CAD build for the part. Positions are in the model's coordinates, mm. Give positions to 0.01 mm unless a question says otherwise; leave off trailing zeros. Order: outer loops, then holes, each group sorted by start corner. A loop starts at its lowest first (then second) coordinate and runs counter-clockwise, first axis right, second up. Notation, with made-up numbers: M 27.25,75.25 L 61.25,75.25 A25 ccw 61.25,102.25 Z; hole C 76.25,23 d4. An arc over 180 degrees is marked long. Put each result on its own line as item: value. Start each with the question number.
1) Cut at C-C (x = 35). Write the cut outline in (y, z).
2) Cut at D-D (y = -9.5). Write the cut outline in (x, z).
3) Drill centre lines: line 1 (Z direction, x = 22, y = -15.5); line 2 (Z direction, x = -30, y = -5); line 3 (Y direction, x = -48, z = -21.5). Where is each one in solid material? Low to high. Write a range as [from, to].
4) Cut at B-B (y = -20). Write the cut outline in (x, z), and give its area (3 significant figures).
5) Pin check, flat tips, straight feed: pin 1 (6 mm diameter, centred on x = -36.5, z = -24, fed in from +Y); pin 2 (0.8 mm diameter, centred on y = 0, z = 15, fed in from -X); pin 3 (12 mm diameter, centred on x = -32.5, y = -9, fed in from +Z). Stop position of each tip, or through.
6) Cut at A-A (z = -14). Write the cut outline in (x, y), and give its area (3 significant figures).
```python
from build123d import *

# Parameters (mm, degrees)
F0_R     = 12.7
F1_DEPTH = 38.5
F2_DEPTH = 23.11
F3_DEPTH = 6.5


with BuildPart() as f1:
    # F0 (on Top) → F1 (new body)
    with BuildSketch(Plane.XY):
        with BuildLine():
            Line((53.5, -25), (53.5, 25))
            Line((53.5, 25), (-28.5, 25))
            ThreePointArc((-28.5, 25), (-46.1776695297, 17.6776695297), (-53.5, 0))
            Line((-53.5, 0), (-53.5, -25))
            Line((-53.5, -25), (53.5, -25))
        make_face()
        with Locations((-28.5, 0)):
            Circle(F0_R, mode=Mode.SUBTRACT)
        with Locations((-28.5, 0)):
            Circle(F0_R)
        with BuildLine():
            ThreePointArc((-31.6598892386, 0.76), (-28.117338286, 3.2273936873), (-25.25, 0))
            ThreePointArc((-25.25, 0), (-28.117338286, -3.2273936873), (-31.6598892386, -0.76))
            ThreePointArc((-31.6598892386, -0.76), (-31.75, 0), (-31.6598892386, 0.76))
        make_face(mode=Mode.SUBTRACT)
        with BuildLine():
            ThreePointArc((-31.6598892386, -0.76), (-28.117338286, -3.2273936873), (-25.25, 0))
            ThreePointArc((-25.25, 0), (-28.117338286, 3.2273936873), (-31.6598892386, 0.76))
            Line((-31.6598892386, 0.76), (-31.1098892386, 0.76))
            Line((-31.1098892386, 0.76), (-31.1098892386, -0.76))
            Line((-31.1098892386, -0.76), (-31.6598892386, -0.76))
        make_face()
        with BuildLine():
            Line((-31.1098892386, 0.76), (-31.6598892386, 0.76))
            ThreePointArc((-31.6598892386, 0.76), (-31.75, 0), (-31.6598892386, -0.76))
            Line((-31.6598892386, -0.76), (-31.1098892386, -0.76))
            Line((-31.1098892386, -0.76), (-31.1098892386, 0.76))
        make_face()
    extrude(amount=-F1_DEPTH)

    # F0 (on Top) → F2 (join)
    with BuildSketch(Plane.XY):
        with BuildLine():
            ThreePointArc((-31.6598892386, -0.76), (-28.117338286, -3.2273936873), (-25.25, 0))
            ThreePointArc((-25.25, 0), (-28.117338286, 3.2273936873), (-31.6598892386, 0.76))
            Line((-31.6598892386, 0.76), (-31.1098892386, 0.76))
            Line((-31.1098892386, 0.76), (-31.1098892386, -0.76))
            Line((-31.1098892386, -0.76), (-31.6598892386, -0.76))
        make_face()
    extrude(amount=F2_DEPTH)

    # F0 (on Top) → F3 (join)
    with BuildSketch(Plane.XY):
        with Locations((-28.5, 0)):
            Circle(F0_R)
        with BuildLine():
            ThreePointArc((-31.6598892386, 0.76), (-28.117338286, 3.2273936873), (-25.25, 0))
            ThreePointArc((-25.25, 0), (-28.117338286, -3.2273936873), (-31.6598892386, -0.76))
            ThreePointArc((-31.6598892386, -0.76), (-31.75, 0), (-31.6598892386, 0.76))
        make_face(mode=Mode.SUBTRACT)
        with BuildLine():
            Line((-31.1098892386, 0.76), (-31.6598892386, 0.76))
            ThreePointArc((-31.6598892386, 0.76), (-31.75, 0), (-31.6598892386, -0.76))
            Line((-31.6598892386, -0.76), (-31.1098892386, -0.76))
            Line((-31.1098892386, -0.76), (-31.1098892386, 0.76))
        make_face()
    extrude(amount=F3_DEPTH)


solid = f1.part
```
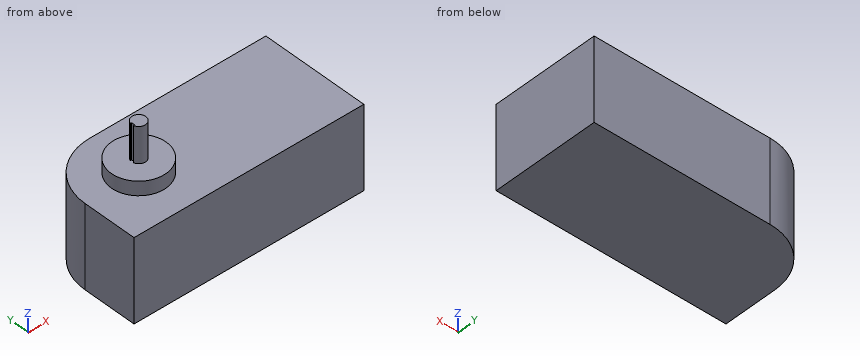
Solution:
1. outline: M -25,-38.5 L 25,-38.5 L 25,0 L -25,0 Z
2. outline: M -53.5,-38.5 L 53.5,-38.5 L 53.5,0 L -20.07,0 L -20.07,6.5 L -36.93,6.5 L -36.93,0 L -53.5,0 Z
3. line 1: [-38.5, 0]
3. line 2: [-38.5, 6.5]
3. line 3: [-25, 15.64]
4. outline: M -53.5,-38.5 L 53.5,-38.5 L 53.5,0 L -53.5,0 Z
4. area: 4,120 mm²
5. pin 1: y = 24.49
5. pin 2: x = -31.11
5. pin 3: z = 6.5
6. outline: M -53.5,-25 L 53.5,-25 L 53.5,25 L -28.5,25 A25 ccw -53.5,0 Z
6. area: 5,220 mm²
